Input: dimensioned drawing with shaded views. Units: mm. Origin: part minimum x, y, z. Round coordinates to 2 decimals unless told otherwise and drop trailing zeros. Write each loop counter-clockwise with the first axis right and the second up, starting at its lowest first coordinate (ties: lowest second). Pieces come first, ordered by that corner, then holes. Notation, with made-up numbers: M -3.5,-11 L 20.5,-11 A13 ccw 20.5,-3 Z; hole C 57,34 d4. An arc over 180 degrees is marked long. Put each result on its own line as item: value. Start each with the question number.
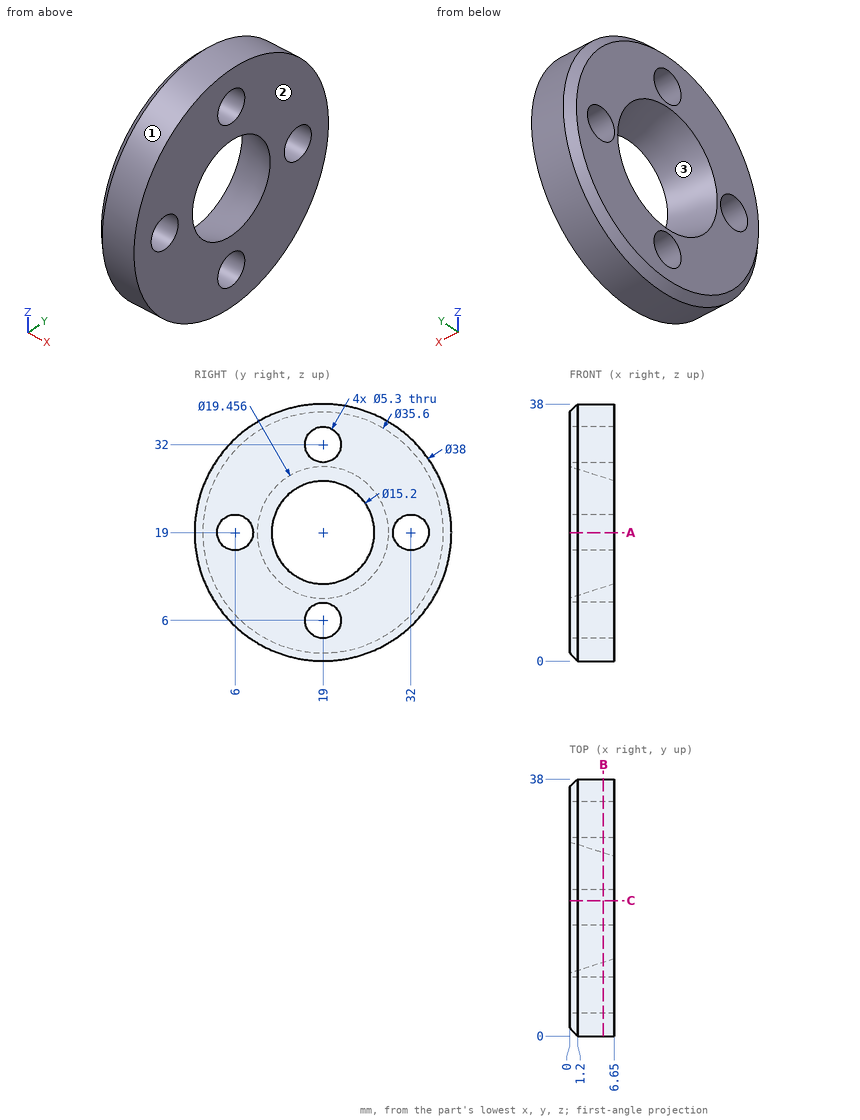
1) Section A-A, the plane z = 19. Output: boundary loops of the cut face in (x, y), and give its area (3 significant figures).
2) Section B-B, the plane x = 5. Output: boundary loops of the cut face in (y, z).
3) Draft query along Y for the marked faces 1, 2 and 3. Return one class per face: +Y half, -Y half, draft (parallel to the pull), parting line (faces both ways), or undercut.
4) Ray query, probe 1 along Z at (x, y) = (0.75, 19); probe 2 along Y at (x, z) = (1.75, 20.5); probe 3 along Y at (x, z) = (2.5, 20). Return the intervals inside material, ascending.
5) Section C-C, the plane y = 20. Give the number of separate pieces and of enclosed holes in the cut face, and give its area (3 significant figures).
6) First-contact query: pin 1 (1 mm diameter, centred on x = 4, y = 23.5, fed in from +Z). Flat tip, straight axial feed; report the tip coordinate or a pass-through.
Solved:
1. outline: M 0,1.2 L 1.2,0 L 6.65,0 L 6.65,3.35 L 0,3.35 Z; M 0,8.65 L 6.65,8.65 L 6.65,11.4 L 0,9.27 Z; M 0,28.73 L 6.65,26.6 L 6.65,29.35 L 0,29.35 Z; M 0,34.65 L 6.65,34.65 L 6.65,38 L 1.2,38 L 0,36.8 Z
1. area: 65.5 mm2
2. outline: C 19,19 d38; hole C 6,19 d5.3; hole C 19,19 d16.26; hole C 19,6 d5.3; hole C 19,32 d5.3; hole C 32,19 d5.3
3. face 1: parting line
3. face 2: draft
3. face 3: undercut
4. probe 1: z = 0.45 to 3.35, 8.65 to 9.51, 28.49 to 29.35, 34.65 to 37.55
4. probe 2: y = 0.06 to 3.82, 8.18 to 9.96, 28.04 to 29.82, 34.18 to 37.94
4. probe 3: y = 0.03 to 3.55, 8.45 to 10.13, 27.87 to 29.55, 34.45 to 37.97
5. separate pieces: 4
5. enclosed holes: 0
5. area: 71.2 mm2
6. pin 1: stops at z = 37.57
